Input: part model. Units: mm. Frame: model coordinates. A direction names the side the tool comes from. Coordinates: 2 decimals unless noted, no trailing zeros. Order: outer loops, then holes, each group sorted by start corner. A loop starts at its lowest first (then second) coordinate and runs counter-clockwise, first axis right, second up. Notation, with made-up numbers: (-28.75, 41) -> (-2.75, 41) arc R11 ccw to (-2.75, 52) -> close; hole circle Ø11 at (4, 86). An arc over 180 degrees is marked (long way). Write each question's results on one line, items separated by ' | '.
```python
from build123d import *

# Parameters (mm, degrees)
F0_R     = 52.5
F0_R_2   = 28.575
F1_DEPTH = 60
F2_SIZE  = 1.5
F4_START = 45
F3_R     = 3
F4_DEPTH = 10


with BuildPart() as f1:
    # F0 (on Front) → F1 (new body)
    with BuildSketch(Plane.XZ):
        Circle(F0_R)
        Circle(F0_R_2, mode=Mode.SUBTRACT)
    extrude(amount=F1_DEPTH)

    # F2
    f2_edges = [f1.edges().sort_by_distance(p)[0] for p in [
        (-52.5, -60, 0),
        (-28.575, -60, 0),
        (-52.5, 0, 0),
        (-28.575, 0, 0),
    ]]
    chamfer(f2_edges, length=F2_SIZE)

    # F3 (on Right) → F4 (cut)
    with BuildSketch(Plane.YZ.offset(F4_START)):
        with Locations((-30, 0)):
            Circle(F3_R)
    extrude(amount=F4_DEPTH, mode=Mode.SUBTRACT)


solid = f1.part
```
(1) Cut plane B-B, the plane z = 0. Return loops of the section in (x, y) (3 decimals), plus the area to 3 significant figures.
Return value:
outline: (-52.5, -58.5) -> (-51, -60) -> (-30.075, -60) -> (-28.575, -58.5) -> (-28.575, -1.5) -> (-30.075, 0) -> (-51, 0) -> (-52.5, -1.5) -> close; (28.575, -58.5) -> (30.075, -60) -> (51, -60) -> (52.5, -58.5) -> (52.5, -33) -> (45, -33) -> (45, -27) -> (52.5, -27) -> (52.5, -1.5) -> (51, 0) -> (30.075, 0) -> (28.575, -1.5) -> close | area: 2,820 mm2
(2) Pin query (flat end, axial travel): P1, Ø1, axis at x = 40.5, y = -49, coming from the -Z side; P2, Ø5.5, axis at y = -30, z = 0, coming from the +X side; P3, Ø5, axis at x = 31, y = -9.5, coming from the +Z side. Return the tip coordinate at first contact, or that it passes through.
Return value:
P1: z = -34 | P2: x = 45 | P3: z = 44.09
(3) Cut plane C-C, the plane y = -21. Return loops of the section in (x, z) (3 decimals).
Return value:
outline: circle Ø105 at (0, 0); hole circle Ø57.15 at (0, 0)
(4) Line query: line 1 along Y through (x, z) = (48, 0); line 2 along Z through (x, y) = (0, -45) (3 decimals); line 3 along X through (y, z) = (-21.5, 0.5). Output: solid intervals per line, ascending. Write a range as from..to.
Return value:
line 1: -60..-33, -27..0 | line 2: -52.5..-28.575, 28.575..52.5 | line 3: -52.5..-28.57, 28.57..52.5
(5) Mould query, pull axis Z, two halves, no side actions, for faces 1 (the face through (49, -33, 0)), 2 (the face through (50.076, -29.601, 15.77)), 3 (the face through (22, -60, -22)). Classes: +Z half, -Z half, draft (parallel to the pull), parting line (faces both ways), or undercut.
Return value:
face 1: undercut | face 2: parting line | face 3: draft
(6) Reachability of faces 4 (the face through (22, 0, -22)), 5 (the face through (45, -30, 0)) from +Z, -Z, +X, -X, +Y, -Y: full face, straight path, thin tool, end or side. Return the list, or none.
Return value:
face 4: +Z, -Z, +X, -X, +Y | face 5: +X
(7) Cut plane A-A, the plane x = 0. Return loops of the section in (y, z) (3 decimals), plus the area to 3 significant figures.
Return value:
outline: (-60, -51) -> (-58.5, -52.5) -> (-1.5, -52.5) -> (0, -51) -> (0, -30.075) -> (-1.5, -28.575) -> (-58.5, -28.575) -> (-60, -30.075) -> close; (-60, 30.075) -> (-58.5, 28.575) -> (-1.5, 28.575) -> (0, 30.075) -> (0, 51) -> (-1.5, 52.5) -> (-58.5, 52.5) -> (-60, 51) -> close | area: 2,860 mm2
(8) Cut plane D-D, the plane y = -30. Return loops of the section in (x, z) (3 decimals), plus the area to 3 significant figures.
Return value:
outline: (45, -3) -> (45, 3) -> (52.414, 3) arc R52.5 ccw (long way) to (52.414, -3) -> close; hole circle Ø57.15 at (0, 0) | area: 6,050 mm2
